```python
from build123d import *

# Parameters (mm, degrees)
ESBO_O1_R                = 1.5
RESSALTO_EXTRUS_O1_DEPTH = 3


with BuildPart() as part:
    # Esboço1 → Ressalto-extrusão1 (new body)
    with BuildSketch(Plane(origin=(0, 0, 0), x_dir=(1, 0, 0), z_dir=(0, 1, 0))):
        with BuildLine():
            Line((-2.838975028, -25.45488959), (-1.5, -33.95488959))
            ThreePointArc((-1.5, -33.95488959), (0, -35.556863977), (1.5, -33.95488959))
            Line((1.5, -33.95488959), (2.838975028, -25.45488959))
            ThreePointArc((2.838975028, -25.45488959), (5.508963035, -3.818784756), (6.499428658, 17.958929684))
            ThreePointArc((6.499428658, 17.958929684), (6.499717622, 18.002020025), (6.5, 18.04511041))
            ThreePointArc((6.5, 18.04511041), (0, 24.54511041), (-6.5, 18.04511041))
            ThreePointArc((-6.5, 18.04511041), (-6.499717622, 18.002020025), (-6.499428658, 17.958929683))
            ThreePointArc((-6.499428658, 17.958929683), (-5.508963035, -3.818784756), (-2.838975028, -25.45488959))
        make_face()
        with Locations(Location((0, -25.45488959, 0), (0, 0, 270))):
            Circle(ESBO_O1_R, mode=Mode.SUBTRACT)
        Polygon((-1.5, -10.95488959), (0, -10.95488959), (1.5, -10.95488959), (1.5, -20.95488959), (0, -20.95488959), (-1.5, -20.95488959), align=None, mode=Mode.SUBTRACT)
        with Locations(Location((0, -6.45488959, 0), (0, 0, 270))):
            Circle(ESBO_O1_R, mode=Mode.SUBTRACT)
        with Locations(Location((0, 18.04511041, 0), (0, 0, 270))):
            Circle(ESBO_O1_R, mode=Mode.SUBTRACT)
    extrude(amount=RESSALTO_EXTRUS_O1_DEPTH)


solid = part.part
```
CAD build for the part. Positions are in the model's coordinates, mm. A direction names the side the tool comes from. Coordinates: 2 decimals unless noted, no trailing zeros. Write each loop counter-clockwise with the first axis right and the second up, starting at its lowest first coordinate (ties: lowest second). Pieces come first, ordered by that corner, then holes. Notation, with made-up numbers: (29, 45.25) -> (33, 45.25) arc R26 cw to (33, 80.25) -> close; hole circle Ø11 at (58.25, 87.25). An arc over 180 degrees is marked (long way). Return JSON: item names as keys, results as strings. Group by question number.
Q1. Flat gauge pins, fed straight in: pin 1 (2.5 mm diameter, centred on x = 0, z = 6.45, fed in from -Y); pin 2 (1.5 mm diameter, centred on y = 1.5, z = -11, fed in from -X); pin 3 (0.9 mm diameter, centred on y = 1, z = 16, fed in from +X). Where does each tip first touch, or does it go through?
Q2. Drill centre lines: line 1 (X direction, y = 1.1, z = 7.5); line 2 (X direction, y = 1.45, z = 13.5); line 3 (X direction, y = 1.25, z = -11.5). Where is each one in solid material? Low to high.
Q3. Which spindle directions (+Z, -Z, +X, -X, +Y, -Y) get a long thin tool onto all of the face, cutting with end or side? Do faces 1 (the face through (0, 1, 10.955)), 2 (the face through (5.483, 1.479, 4.123)). Say none if no direction does.
Q4. Cut at B-B, the plane y = 0.45. Give the cut face in (x, z).
Q5. Cut at D-D, the plane z = 31. Give the cut face in (x, y), then the cut area to 3 significant figures.
Q6. Cut at A-A, the plane x = 0. Give the cut face in (y, z), then the cut area to 3 significant figures.
Q7. Cut at C-C, the plane z = 7. Give the cut face in (x, y), then the cut area to 3 significant figures.
Returned:
{
 "1": {"pin 1": "passes through", "pin 2": "stops at x = -6.39", "pin 3": "stops at x = 4.27"},
 "2": {"line 1": "x = -5.17 to -1.08, 1.08 to 5.17", "line 2": "x = -4.52 to -1.5, 1.5 to 4.52", "line 3": "x = -6.38 to 6.38"},
 "3": {"face 1": "+Y, -Y", "face 2": "+Z, +X, +Y, -Y"},
 "4": {"outline": "(-6.5, -18.05) arc R6.5 ccw to (6.5, -18.05) arc R281.93 ccw to (6.5, -17.96) arc R281.97 ccw to (2.84, 25.45) -> (1.5, 33.95) arc R1.5 ccw (long way) to (-1.5, 33.95) -> (-2.84, 25.45) arc R281.97 ccw to (-6.5, -17.96) arc R281.93 ccw to start; hole circle Ø3 at (0, -18.05); hole circle Ø3 at (0, 6.45); hole (-1.5, 10.95) -> (1.5, 10.95) -> (1.5, 20.95) -> (-1.5, 20.95) -> close; hole circle Ø3 at (0, 25.45)"},
 "5": {"outline": "(-1.97, 0) -> (1.97, 0) -> (1.97, 3) -> (-1.97, 3) -> close", "area": "11.8 mm2"},
 "6": {"outline": "(0, -24.55) -> (3, -24.55) -> (3, -19.55) -> (0, -19.55) -> close; (0, -16.55) -> (3, -16.55) -> (3, 4.95) -> (0, 4.95) -> close; (0, 7.95) -> (3, 7.95) -> (3, 10.95) -> (0, 10.95) -> close; (0, 20.95) -> (3, 20.95) -> (3, 23.95) -> (0, 23.95) -> close; (0, 26.95) -> (3, 26.95) -> (3, 35.56) -> (0, 35.56) -> close", "area": "123 mm2"},
 "7": {"outline": "(-5.22, 0) -> (-1.4, 0) -> (-1.4, 3) -> (-5.22, 3) -> close; (1.4, 0) -> (5.22, 0) -> (5.22, 3) -> (1.4, 3) -> close", "area": "23.0 mm2"}
}
